Source: CAD feature listing. Evaluate the final solid. Frame: model axes, mm. A direction names the side the tool comes from. Round coordinates to 2 decimals unless told otherwise and drop trailing zeros. Loops run counter-clockwise (first coordinate to the right, second up) from the corner with the lowest first, then second, coordinate; pieces in that order, holes last. Notation, with made-up numbers: (6, 76) -> (22, 76) arc R6 cw to (22, 83) -> close; hole circle Ø6 at (47, 77.25). An arc over 180 degrees is marked (long way). Write item = value, one per line.
from build123d import *

# Parameters (mm, degrees)
F0_W     = 331
F0_H     = 218
F1_DEPTH = 9
F2_W     = 299
F2_H     = 176
F3_DEPTH = 1
F4_R     = 3
F5_DEPTH = 2
F6_R     = 5
F6_R_2   = 2
F7_DEPTH = 135.5
F8_R     = 5
F9_R     = 1


with BuildPart() as f1:
    # F0 (on Front) → F1 (new body)
    with BuildSketch(Plane.XZ):
        with Locations((0, 109)):
            Rectangle(F0_W, F0_H)
    extrude(amount=F1_DEPTH)

    # F2 (on face) → F3 (cut)
    with BuildSketch(Plane.XZ.offset(9)):
        with Locations((0, 112)):
            Rectangle(F2_W, F2_H)
    extrude(amount=-F3_DEPTH, mode=Mode.SUBTRACT)

    # F4 (on face) → F5 (cut)
    with BuildSketch(Plane.XZ.offset(9)):
        with Locations((0, 209)):
            Circle(F4_R)
    extrude(amount=-F5_DEPTH, mode=Mode.SUBTRACT)

    # F6 (on Right) → F7 (join, symmetric)
    with BuildSketch(Plane.YZ):
        with Locations((-9, -4)):
            Circle(F6_R)
        with Locations((-9, -4)):
            Circle(F6_R_2, mode=Mode.SUBTRACT)
    extrude(amount=F7_DEPTH, both=True)

    # F8
    f8_edges = [f1.edges().sort_by_distance(p)[0] for p in [
        (165.5, -4.5, 0),
        (165.5, -4.5, 218),
        (-165.5, -4.5, 218),
        (-165.5, -4.5, 0),
    ]]
    fillet(f8_edges, radius=F8_R)

    # F9
    f9_edges = [f1.edges().sort_by_distance(p)[0] for p in [
        (-165.5, -9, 109),
        (-165.5, 0, 109),
    ]]
    fillet(f9_edges, radius=F9_R)


solid = f1.part
1. Section query B-B (x = 39.5). Return the cut outline in (y, z), then the cut area to 3 significant figures.
Evaluation:
outline = (-9, 1) arc R5 ccw (long way) to (-6, 0) -> (-1, 0) arc R1 ccw to (0, 1) -> (0, 217) arc R1 ccw to (-1, 218) -> (-8, 218) arc R1 ccw to (-9, 217) -> (-9, 200) -> (-8, 200) -> (-8, 24) -> (-9, 24) -> close; hole circle Ø4 at (-9, -4)
area = 1,850 mm²
2. Section query A-A (z = 75). Return the cut outline in (x, y).
Evaluation:
outline = (-165.5, -8) arc R1 ccw to (-164.5, -9) -> (-149.5, -9) -> (-149.5, -8) -> (149.5, -8) -> (149.5, -9) -> (164.5, -9) arc R1 ccw to (165.5, -8) -> (165.5, -1) arc R1 ccw to (164.5, 0) -> (-164.5, 0) arc R1 ccw to (-165.5, -1) -> close
3. Contact query for flat-ended pins moving along their axis: pin 1 Ø0.5 at (x, y) = (-65, -8.5) entering from +Z; pin 2 Ø8 at (y, z) = (-7.5, -3) entering from -X; pin 3 Ø10 at (x, z) = (-123.5, 82.5) entering from -Y; pin 4 Ø1.1 at (y, z) = (-8.5, 92.5) entering from -X. Output: stop coordinate, or through.
Evaluation:
pin_1 = 217.97
pin_2 = -163.5
pin_3 = -8
pin_4 = -165.5
4. Line query: probe 1 along X at (y, z) = (-7.4, 209); probe 2 along Y at (x, z) = (142, 183); probe 3 along Y at (x, z) = (-17, 6). Output: solid intervals per line, ascending. Write a range as from..to.
Evaluation:
probe_1 = -165.5..-3, 3..165.5
probe_2 = -8..0
probe_3 = -9..0
5. Set-up query: faces 1 (the face through (11, -9, 22)), 2 (the face through (-2, 0, 111)). Return all of +Z, -Z, +X, -X, +Y, -Y with unobstructed straight access to the full face (end or side cutting, diameter ignored); none if empty.
Evaluation:
face_1 = +Z, +X, -X, -Y
face_2 = +Z, -Z, +X, -X, +Y
6. Mould query, pull axis Z, two halves, no side actions, for faces 3 (the face through (-2, -8, 113)), 4 (the face through (-2, -4, 218)), 5 (the face through (-165.5, -4, 108)). Classes: released by +Z, released by -Z, zero draft, split by the parting line, or undercut.
Evaluation:
face_3 = undercut
face_4 = released by +Z
face_5 = zero draft
